Work out the finished part from the listing and answer in its coordinate system (mm). Round coordinates to 2 decimals unless told otherwise and drop trailing zeros. Loops run counter-clockwise (first coordinate to the right, second up) from the corner with the lowest first, then second, coordinate; pieces in that order, holes last. Notation, with made-up numbers: (63.25, 72) -> (115.25, 72) arc R8 ccw to (115.25, 76) -> close; hole circle Ø4 at (49, -30). An arc over 180 degrees is marked (long way). Use CSV: the item, a comma, the result in double quotes. Start each with the question number.
from build123d import *

# Parameters (mm, degrees)
SKETCH1_W           = 74
SKETCH1_H           = 42
SKETCH1_R           = 1.6
SKETCH1_W_2         = 36
SKETCH1_H_2         = 30
BOSS_EXTRUDE1_DEPTH = 1.25
FILLET1_R           = 10


with BuildPart() as part:
    # Sketch1 → Boss-Extrude1 (new body)
    with BuildSketch(Plane(origin=(0, 0, 0), x_dir=(1, 0, 0), z_dir=(0, 1, 0))):
        Rectangle(SKETCH1_W, SKETCH1_H)
        with Locations(Location((-33, 0, 0), (0, 0, 270))):
            Circle(SKETCH1_R, mode=Mode.SUBTRACT)
        with Locations(Location((33, 0, 0), (0, 0, 90))):
            Circle(SKETCH1_R, mode=Mode.SUBTRACT)
        Rectangle(SKETCH1_W_2, SKETCH1_H_2, mode=Mode.SUBTRACT)
    extrude(amount=BOSS_EXTRUDE1_DEPTH)

    # Fillet1
    fillet1_edges = [part.edges().sort_by_distance(p)[0] for p in [
        (37, 0.625, 21),
        (-37, 0.625, 21),
        (-37, 0.625, -21),
        (37, 0.625, -21),
    ]]
    fillet(fillet1_edges, radius=FILLET1_R)


solid = part.part
Q1. Section B-B, the plane z = -9 is taken. Write down the section's boundary in (x, y), and give its area (3 significant figures).
Q2. For a pull along Z with two mould halves and no side action, classify faces 1 (the cylindrical face through (-34.42, 0.62, 0.74)), 2 (the cylindrical face through (-34.15, 0.63, -17.99)), 3 (the cylindrical face through (33.99, 0.63, 18.15)) as pulls with the +Z half, pulls with the -Z half, needs draft (parallel to the pull), parting line crosses it, or undercut.
Q3. Straight lines are drawn through the part: line 1 (X direction, y = 0.3, z = 0); line 2 (Z direction, x = -12, y = 0.8); line 3 (X direction, y = 1, z = 9). For each, find the intervals that lie inside material, in ascending order. Write a range as from..to.
Q4. Each of these flat-tipped pins is pushed along its axis until it touches: pin 1 (3.5 mm diameter, centred on x = -33, z = 0, fed in from +Y); pin 2 (2 mm diameter, centred on x = 16, z = -5, fed in from +Y). Where does it stop, or does it pass through?
Q5. Section A-A, the plane y = 0.2 is taken. Write down the section's boundary in (x, z), and give its area (3 significant figures).
Q6. Section C-C, the plane x = -4 is taken. Write down the section's boundary in (y, z).
Q7. Section D-D, the plane z = -17 is taken. Write down the section's boundary in (x, y).
Report:
1,outline,"(-37, 0) -> (-18, 0) -> (-18, 1.25) -> (-37, 1.25) -> close; (18, 0) -> (37, 0) -> (37, 1.25) -> (18, 1.25) -> close"
1,area,"47.5 mm²"
2,face 1,"undercut"
2,face 2,"pulls with the -Z half"
2,face 3,"pulls with the +Z half"
3,line 1,"x = -37..-34.6, -31.4..-18, 18..31.4, 34.6..37"
3,line 2,"z = -21..-15, 15..21"
3,line 3,"x = -37..-18, 18..37"
4,pin 1,"stops at y = 1.25"
4,pin 2,"passes through"
5,outline,"(-37, -11) arc R10 ccw to (-27, -21) -> (27, -21) arc R10 ccw to (37, -11) -> (37, 11) arc R10 ccw to (27, 21) -> (-27, 21) arc R10 ccw to (-37, 11) -> close; hole circle Ø3.2 at (-33, 0); hole (-18, -15) -> (18, -15) -> (18, 15) -> (-18, 15) -> close; hole circle Ø3.2 at (33, 0)"
5,area,"1,930 mm²"
6,outline,"(0, -21) -> (1.25, -21) -> (1.25, -15) -> (0, -15) -> close; (0, 15) -> (1.25, 15) -> (1.25, 21) -> (0, 21) -> close"
7,outline,"(-35, 0) -> (35, 0) -> (35, 1.25) -> (-35, 1.25) -> close"
